Work out the finished part from the listing and answer in its coordinate system (mm). Round coordinates to 2 decimals unless told otherwise and drop trailing zeros. Write each loop counter-clockwise with the first axis right and the second up, starting at its lowest first coordinate (ties: lowest second). Pieces come first, ordered by that corner, then holes. Notation, with made-up numbers: (6, 3.5) -> (60, 3.5) arc R22 cw to (60, 37.5) -> close; hole circle Ø10 at (-0.5, 30). An arc over 180 degrees is marked (long way). Answer as a JSON object with one key per item and string values. Group by question number.
from build123d import *

# Parameters (mm, degrees)
CROQUIS3_R              = 9.54
CROQUIS3_R_2            = 1.825
CROQUIS3_W              = 8.4
CROQUIS3_H              = 4.2
CROQUIS3_W_2            = 4.2
CROQUIS3_H_2            = 8.4
SALIENTE_EXTRUIR1_DEPTH = 5


with BuildPart() as part:
    # Croquis3 → Saliente-Extruir1 (new body)
    with BuildSketch(Plane(origin=(0, 0, 0), x_dir=(1, 0, 0), z_dir=(0, 1, 0))):
        with BuildLine():
            Line((50.5587, 0), (76.2, 0))
            ThreePointArc((76.2, 0), (0, -35.242297755), (-76.2, 0))
            Line((-76.2, 0), (-50.5587, 0))
            Line((-50.5587, 0), (-50.5587, 160))
            ThreePointArc((-50.5587, 160), (0, 174.754698219), (50.5587, 160))
            Line((50.5587, 160), (50.5587, 0))
        make_face()
        with Locations(Location((0, 0, 0), (0, 0, 270))):
            Circle(CROQUIS3_R, mode=Mode.SUBTRACT)
        with Locations(Location((33.5337, 44.7, 0), (0, 0, 270))):
            Circle(CROQUIS3_R_2, mode=Mode.SUBTRACT)
        with Locations(Location((11.5437, 44.7, 0), (0, 0, 90))):
            Circle(CROQUIS3_R_2, mode=Mode.SUBTRACT)
        with Locations(Location((-33.5337, 44.7, 0), (0, 0, 90))):
            Circle(CROQUIS3_R_2, mode=Mode.SUBTRACT)
        with Locations(Location((-11.5437, 44.7, 0), (0, 0, 270))):
            Circle(CROQUIS3_R_2, mode=Mode.SUBTRACT)
        with Locations(Location((24.7337, 22.125, 0), (0, 0, 270))):
            Circle(CROQUIS3_R_2, mode=Mode.SUBTRACT)
        with Locations(Location((-24.7337, 22.125, 0), (0, 0, 90))):
            Circle(CROQUIS3_R_2, mode=Mode.SUBTRACT)
        with Locations((40.8587, 131.7)):
            Rectangle(CROQUIS3_W, CROQUIS3_H, mode=Mode.SUBTRACT)
        with Locations((40.8587, 124.1)):
            Rectangle(CROQUIS3_W, CROQUIS3_H, mode=Mode.SUBTRACT)
        with Locations((40.8587, 139.3)):
            Rectangle(CROQUIS3_W, CROQUIS3_H, mode=Mode.SUBTRACT)
        with Locations((-40.8587, 124.1)):
            Rectangle(CROQUIS3_W, CROQUIS3_H, mode=Mode.SUBTRACT)
        with Locations((-40.8587, 131.7)):
            Rectangle(CROQUIS3_W, CROQUIS3_H, mode=Mode.SUBTRACT)
        with Locations((-40.8587, 139.3)):
            Rectangle(CROQUIS3_W, CROQUIS3_H, mode=Mode.SUBTRACT)
        with Locations((33.9987, 0)):
            Rectangle(CROQUIS3_W_2, CROQUIS3_H_2, mode=Mode.SUBTRACT)
        with Locations((41.5987, 0)):
            Rectangle(CROQUIS3_W_2, CROQUIS3_H_2, mode=Mode.SUBTRACT)
        with Locations((26.3987, 0)):
            Rectangle(CROQUIS3_W_2, CROQUIS3_H_2, mode=Mode.SUBTRACT)
        with Locations((-41.5987, 0)):
            Rectangle(CROQUIS3_W_2, CROQUIS3_H_2, mode=Mode.SUBTRACT)
        with Locations((-33.9987, 0)):
            Rectangle(CROQUIS3_W_2, CROQUIS3_H_2, mode=Mode.SUBTRACT)
        with Locations((-26.3987, 0)):
            Rectangle(CROQUIS3_W_2, CROQUIS3_H_2, mode=Mode.SUBTRACT)
        Polygon((19.3637, 34.2), (19.3637, 41.35), (15.4687, 41.35), (15.4687, 48.05), (19.3637, 48.05), (19.3637, 55.2), (25.7137, 55.2), (25.7137, 48.05), (29.6087, 48.05), (29.6087, 41.35), (25.7137, 41.35), (25.7137, 34.2), align=None, mode=Mode.SUBTRACT)
        Polygon((-19.3637, 34.2), (-19.3637, 41.35), (-15.4687, 41.35), (-15.4687, 48.05), (-19.3637, 48.05), (-19.3637, 55.2), (-25.7137, 55.2), (-25.7137, 48.05), (-29.6087, 48.05), (-29.6087, 41.35), (-25.7137, 41.35), (-25.7137, 34.2), align=None, mode=Mode.SUBTRACT)
    extrude(amount=SALIENTE_EXTRUIR1_DEPTH)


solid = part.part
1) Each of these flat-tipped pins is pushed along its axis until it touches: P1, Ø1.5, axis at y = 2, z = 1, coming from the -X side; P2, Ø1.3, axis at x = -34.5, y = 2, coming from the -Z side; P3, Ø2, axis at y = 2, z = -132, coming from the +X side; P4, Ø12, axis at x = -57.5, z = -73.5, coming from the +Y side. Where does it stop, or does it pass through?
2) Straight lines are drawn through the part: L1, parallel to X at y = 1.55, z = -133; L2, parallel to X at y = 2.5, z = -53; L3, parallel to Z at x = -43, y = 3.3. For each, find the intervals that lie inside material, in ascending order.
3) A cutting plane is placed at C-C on y = 3.15. State how many separate pieces and enclosed holes the cut face has, plus the area to 3 significant figures.
4) A cutting plane is placed at A-A on x = 0. Determine the outline of the cut face in (y, z), plus the area to 3 significant figures.
5) A cutting plane is placed at B-B on z = -81.5. Determine the outline of the cut face in (x, y), plus the area to 3 significant figures.
6) For a pull along X with two mould halves and no side action, classify faces 1 (the face through (-0.75, 2.46, -174.75)), 2 (the face through (-41, 2, -133.8)) as released by +X, released by -X, zero draft, split by the parting line, or undercut.
Established:
{
 "1": {"P1": "stops at x = -75.99", "P2": "stops at z = -168.45", "P3": "stops at x = 50.56", "P4": "passes through"},
 "2": {"L1": "x = -50.56 to -45.06, -36.66 to 36.66, 45.06 to 50.56", "L2": "x = -50.56 to -25.71, -19.36 to 19.36, 25.71 to 50.56", "L3": "z = -164.34 to -141.4, -137.2 to -133.8, -129.6 to -126.2, -122 to -4.2, 4.2 to 25.53"},
 "3": {"separate pieces": "1", "enclosed holes": "21", "area": "19,800 mm²"},
 "4": {"outline": "(0, -174.75) -> (5, -174.75) -> (5, -9.54) -> (0, -9.54) -> close; (0, 9.54) -> (5, 9.54) -> (5, 35.24) -> (0, 35.24) -> close", "area": "955 mm²"},
 "5": {"outline": "(-50.56, 0) -> (50.56, 0) -> (50.56, 5) -> (-50.56, 5) -> close", "area": "506 mm²"},
 "6": {"face 1": "split by the parting line", "face 2": "undercut"}
}
